Build history of the part. All positions in model axes, mm. Give positions to 0.01 mm unless a question says otherwise; leave off trailing zeros. Order: outer loops, then holes, each group sorted by start corner. A loop starts at its lowest first (then second) coordinate and runs counter-clockwise, first axis right, second up. Notation, with made-up numbers: M 60,54 L 119,54 A23 cw 119,69 Z; hole C 36.25,-0.5 d7. An arc over 180 degrees is marked long. Use CSV: the item, a comma, the result in double quotes. Start each with the question number.
Item 1: Band-saw the part on D-D on z = 62. Write the cut outline in (x, y).
Item 2: Band-saw the part on B-B on y = 70.5. Write the cut outline in (x, z), plus the area to 3 significant figures.
Item 3: Pin check, flat tips, straight feed: P1, Ø3.5, axis at x = 5, y = 77.5, coming from the -Z side; P2, Ø1.3, axis at x = 6, z = 62.5, coming from the +Y side; P3, Ø1.2, axis at y = 42.63, z = 42.63, coming from the -X side; P4, Ø4, axis at x = 5, z = 70, coming from the -Y side. Stop position of each tip, or through.
Item 4: Band-saw the part on C-C on z = 147.38. Write the cut outline in (x, y).
Item 5: Band-saw the part on A-A on y = 26.3. Write the cut outline in (x, z).
Item 6: Wall check: line 1 along Z through (x, y) = (7.25, 96); line 2 along Z through (x, y) = (5, 3.9); line 3 along Z through (x, y) = (1.5, 34.5). Give the ranges that are in metal, low to high.
from build123d import *

# Parameters (mm, degrees)
SKETCH_W        = 10
SKETCH_H        = 155
PAD_DEPTH       = 155
SKETCH001_R     = 19.9
SKETCH001_R_2   = 1
POCKET_DEPTH    = 10.001
SKETCH002_R     = 2.2
SKETCH002_W     = 120.5
SKETCH002_H     = 55
POCKET001_DEPTH = 10.001
SKETCH003_R     = 2.2
POCKET002_DEPTH = 10.001
SKETCH004_R     = 2.2
POCKET003_DEPTH = 5
SKETCH005_R     = 2.2
POCKET004_DEPTH = 5
SKETCH006_R     = 2.2
POCKET005_DEPTH = 5
SKETCH007_R     = 26.5
SKETCH007_R_2   = 19.9
POCKET006_DEPTH = 4


with BuildPart() as part:
    # Sketch → Pad (new body)
    with BuildSketch(Plane.XY):
        with Locations((5, 77.5)):
            Rectangle(SKETCH_W, SKETCH_H)
    extrude(amount=PAD_DEPTH)

    # Sketch001 (on Face2 of Pad) → Pocket (cut, through all)
    with BuildSketch(Plane.YZ.offset(10)):
        with Locations((26.3, 26.3)):
            Circle(SKETCH001_R)
        with Locations((128.7, 26.3)):
            Circle(SKETCH001_R)
        with Locations((42.634167, 42.634167)):
            Circle(SKETCH001_R_2)
        with Locations((42.634167, 9.965833)):
            Circle(SKETCH001_R_2)
        with Locations((9.965833, 9.965833)):
            Circle(SKETCH001_R_2)
        with Locations((9.965833, 42.634167)):
            Circle(SKETCH001_R_2)
        with Locations((112.365833, 42.634167)):
            Circle(SKETCH001_R_2)
        with Locations((145.034167, 42.634167)):
            Circle(SKETCH001_R_2)
        with Locations((145.034167, 9.965833)):
            Circle(SKETCH001_R_2)
        with Locations((112.365833, 9.965833)):
            Circle(SKETCH001_R_2)
    extrude(amount=-POCKET_DEPTH, mode=Mode.SUBTRACT)

    # Sketch002 (on Face3 of Pocket) → Pocket001 (cut, through all)
    with BuildSketch(Plane.YZ.offset(10)):
        with Locations((13.17, 86.42)):
            Circle(SKETCH002_R)
        with Locations((140.17, 86.42)):
            Circle(SKETCH002_R)
        with Locations((140.17, 147.38)):
            Circle(SKETCH002_R)
        with Locations((60.25, 122)):
            Rectangle(SKETCH002_W, SKETCH002_H)
    extrude(amount=-POCKET001_DEPTH, mode=Mode.SUBTRACT)

    # Sketch003 (on Face3 of Pocket001) → Pocket002 (cut, through all)
    with BuildSketch(Plane.YZ.offset(10)):
        with Locations((38.75, 70)):
            Circle(SKETCH003_R)
        with Locations((77.5, 70)):
            Circle(SKETCH003_R)
        with Locations((116.25, 70)):
            Circle(SKETCH003_R)
    extrude(amount=-POCKET002_DEPTH, mode=Mode.SUBTRACT)

    # Sketch004 (on Face1 of Pocket002) → Pocket003 (cut)
    with BuildSketch(Plane.XZ):
        with Locations((5, 70)):
            Circle(SKETCH004_R)
        with Locations((5, 62)):
            Circle(SKETCH004_R)
        with Locations((5, 78)):
            Circle(SKETCH004_R)
    extrude(amount=-POCKET003_DEPTH, mode=Mode.SUBTRACT)

    # Sketch005 (on Face9 of Pocket003) → Pocket004 (cut)
    with BuildSketch(Plane(origin=(0, 155, 0), x_dir=(-1, 0, 0), z_dir=(0, 1, 0))):
        with Locations((-5, 78)):
            Circle(SKETCH005_R)
        with Locations((-5, 70)):
            Circle(SKETCH005_R)
        with Locations((-5, 62)):
            Circle(SKETCH005_R)
    extrude(amount=-POCKET004_DEPTH, mode=Mode.SUBTRACT)

    # Sketch006 (on Face2 of Pocket004) → Pocket005 (cut)
    with BuildSketch(Plane(origin=(0, 0, 0), x_dir=(1, 0, 0), z_dir=(0, 0, -1))):
        with Locations((5, -38.75)):
            Circle(SKETCH006_R)
        with Locations((5, -77.5)):
            Circle(SKETCH006_R)
        with Locations((5, -116.25)):
            Circle(SKETCH006_R)
    extrude(amount=-POCKET005_DEPTH, mode=Mode.SUBTRACT)

    # Sketch007 (on Face4 of Pocket005) → Pocket006 (cut)
    with BuildSketch(Plane.YZ.offset(10)):
        with Locations((26.3, 26.3)):
            Circle(SKETCH007_R)
        with Locations((26.3, 26.3)):
            Circle(SKETCH007_R_2, mode=Mode.SUBTRACT)
        with Locations((128.7, 26.3)):
            Circle(SKETCH007_R)
        with Locations((128.7, 26.3)):
            Circle(SKETCH007_R_2, mode=Mode.SUBTRACT)
    extrude(amount=-POCKET006_DEPTH, mode=Mode.SUBTRACT)


solid = part.part
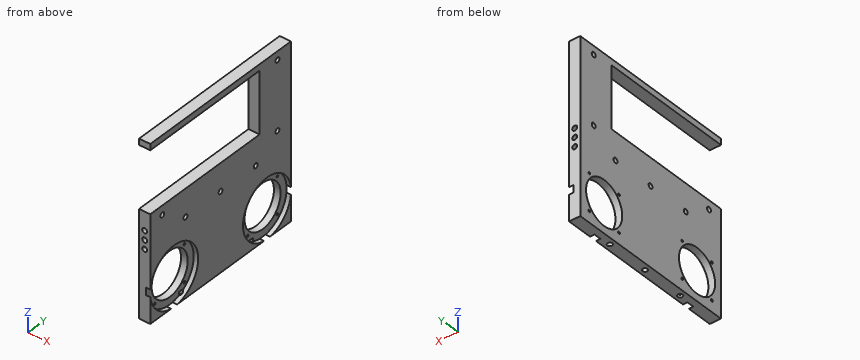
Model answer:
1,outline,"M 0,0 L 2.8,0 L 2.8,5 L 7.2,5 L 7.2,0 L 10,0 L 10,155 L 7.2,155 L 7.2,150 L 2.8,150 L 2.8,155 L 0,155 Z"
2,outline,"M 0,0 L 10,0 L 10,94.5 L 0,94.5 Z; M 0,149.5 L 10,149.5 L 10,155 L 0,155 Z"
2,area,"1,000 mm^2"
3,P1,"stops at z = 5"
3,P2,"stops at y = 150"
3,P3,"passes through"
3,P4,"stops at y = 5"
4,outline,"M 0,120.5 L 10,120.5 L 10,137.97 L 0,137.97 Z; M 0,142.37 L 10,142.37 L 10,155 L 0,155 Z"
5,outline,"M 0,0 L 6,0 L 6,6.4 L 0,6.4 Z; M 0,46.2 L 6,46.2 L 6,52.8 L 10,52.8 L 10,94.5 L 0,94.5 Z; M 0,149.5 L 10,149.5 L 10,155 L 0,155 Z"
6,line 1,"z = 0 to 94.5, 149.5 to 155"
6,line 2,"z = 0 to 59.8, 64.2 to 67.8, 72.2 to 75.8, 80.2 to 94.5, 149.5 to 155"
6,line 3,"z = 0 to 8.17, 44.43 to 94.5, 149.5 to 155"
